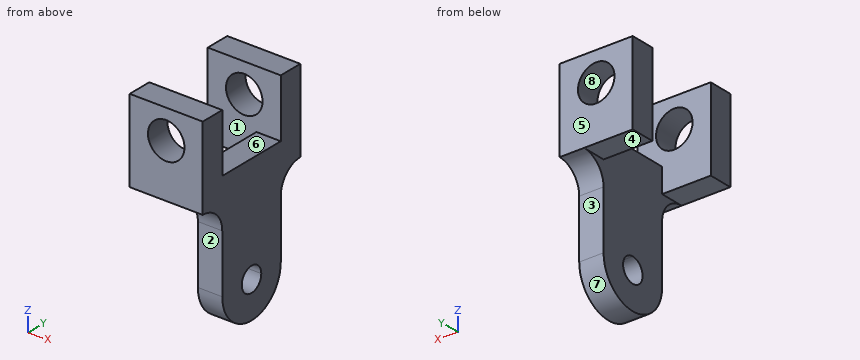
```python
from build123d import *

# Parameters (mm, degrees)
BOSS_EXTRUDE1_DEPTH     = 50
FILLET1_R               = 50
SKETCH2_W               = 150
SKETCH2_H               = 170
BOSS_EXTRUDE2_DEPTH     = 50
SKETCH3_W               = 150
SKETCH3_H               = 170
BOSS_EXTRUDE3_DEPTH     = 50
CUT_EXTRUDE1_DEPTH      = 448.883913531
CUT_EXTRUDE1_DEPTH_BACK = 448.883913531
SKETCH4_R               = 37.5


with BuildPart() as part:
    # Sketch1 → Boss-Extrude1 (new body)
    # profile 1 of 4: a face of its own
    with BuildSketch(Plane.YZ):
        with BuildLine():
            Line((-75, 170), (-75, 0))
            ThreePointArc((-75, 0), (-53.033008589, 53.033008589), (0, 75))
            Line((0, 75), (0, 220))
            Line((0, 220), (-75, 220))
            Line((-75, 220), (-75, 340))
            Line((-75, 340), (-125, 340))
            Line((-125, 340), (-125, 170))
            Line((-125, 170), (-75, 170))
        make_face()
    # profile 2 of 4: a face of its own
    with BuildSketch(Plane.YZ):
        with BuildLine():
            ThreePointArc((0, 75), (53.033008589, 53.033008589), (75, 0))
            Line((75, 0), (75, 170))
            Line((75, 170), (125, 170))
            Line((125, 170), (125, 340))
            Line((125, 340), (75, 340))
            Line((75, 340), (75, 220))
            Line((75, 220), (0, 220))
            Line((0, 220), (0, 75))
        make_face()
    # profile 3 of 4: a face of its own
    with BuildSketch(Plane.YZ):
        with BuildLine():
            ThreePointArc((0, 75), (-53.033008589, 53.033008589), (-75, 0))
            ThreePointArc((-75, 0), (0, -75), (75, 0))
            ThreePointArc((75, 0), (53.033008589, 53.033008589), (0, 75))
        make_face()
        with BuildLine():
            ThreePointArc((25, 0), (-17.67766953, -17.67766953), (0, 25))
            ThreePointArc((0, 25), (17.67766953, 17.67766953), (25, 0))
        make_face(mode=Mode.SUBTRACT)
    # profile 4 of 4: a face of its own
    with BuildSketch(Plane.YZ):
        with BuildLine():
            ThreePointArc((0, 75), (-53.033008589, 53.033008589), (-75, 0))
            ThreePointArc((-75, 0), (0, -75), (75, 0))
            ThreePointArc((75, 0), (53.033008589, 53.033008589), (0, 75))
        make_face()
        with BuildLine():
            ThreePointArc((25, 0), (-17.67766953, -17.67766953), (0, 25))
            ThreePointArc((0, 25), (17.67766953, 17.67766953), (25, 0))
        make_face(mode=Mode.SUBTRACT)
    extrude(amount=-BOSS_EXTRUDE1_DEPTH)

    # Fillet1
    fillet1_edges = [part.edges().sort_by_distance(p)[0] for p in [
        (-25, 75, 170),
        (-25, -75, 170),
    ]]
    fillet(fillet1_edges, radius=FILLET1_R - 0.0001)  # a hair under: the kernel refuses the full size

    # Sketch2 → Boss-Extrude2 (add)
    with BuildSketch(Plane(origin=(0, 125, 0), x_dir=(-1, 0, 0), z_dir=(0, 1, 0))):
        with Locations((75, 255)):
            Rectangle(SKETCH2_W, SKETCH2_H)
    extrude(amount=-BOSS_EXTRUDE2_DEPTH)

    # Sketch3 → Boss-Extrude3 (add)
    with BuildSketch(Plane.XZ.offset(125)):
        with Locations((-75, 255)):
            Rectangle(SKETCH3_W, SKETCH3_H)
    extrude(amount=-BOSS_EXTRUDE3_DEPTH)

    # Sketch4 → Cut-Extrude1 (cut, two sides: drawn at the far end of the back side and taken through both)
    with BuildSketch(Plane.XZ.offset(125).offset(-CUT_EXTRUDE1_DEPTH_BACK)):
        with Locations(Location((-75, 280, 0), (0, 0, 270))):
            Circle(SKETCH4_R)
    extrude(amount=CUT_EXTRUDE1_DEPTH + CUT_EXTRUDE1_DEPTH_BACK, mode=Mode.SUBTRACT)


solid = part.part
```
For this review, take the finished solid that the model builds, in its own axes (mm). Face numbers are marked on the shaded views. A direction names the side the tool comes from. Coordinates: 2 decimals unless noted, no trailing zeros. Loops run counter-clockwise (first coordinate to the right, second up) from the corner with the lowest first, then second, coordinate; pieces in that order, holes last.
1. Add section B-B, the plane x = -75. Give the boundary of the cut face in (y, z).
2. Insertion check: P1, Ø4, axis at x = -35, z = 144.5, coming from the -Y side; P2, Ø12, axis at x = -19.5, y = -12, coming from the -Z side; P3, Ø25, axis at x = -24, z = 45, coming from the +Y side; P4, Ø6, axis at y = -27.5, z = 120.5, coming from the +X side. Each pin has a flat end and moves straight along its axis. Give the tip position at first contact, or say it passes through.
3. For line 1 (X direction, y = 114, z = 280); line 2 (Y direction, x = -120, z = 275); line 3 (Z direction, x = -14, y = 0), list the stretches that pass through material, from the lowest coordinate up.
4. Add section C-C, the plane y = -91. Give the boundary of the cut face in (x, z), then the cut area to 3 significant figures.
5. Mouldability with a two-part tool opening along Y and no side actions: class the marked faces 5, 6, 7 and 8 as +Y half, -Y half, draft (parallel to the pull), parting line (faces both ways), or undercut.
6. Add section D-D, the plane z = 189. Give the boundary of the cut face in (x, y).
7. Add section A-A, the plane z = 280. Give the boundary of the cut face in (x, y), then the cut area to 3 significant figures.
8. For the marked faces 1, 2, 3 and 4, list the 3-axis set-ups (+Z, -Z, +X, -X, +Y, -Y) from which the entire face can be reached by the end or side of a thin tool; tool diameter is ignored.
Result:
1. outline: (-125, 170) - (-75, 170) - (-75, 242.5) - (-125, 242.5) - close; (-125, 317.5) - (-75, 317.5) - (-75, 340) - (-125, 340) - close; (75, 170) - (125, 170) - (125, 242.5) - (75, 242.5) - close; (75, 317.5) - (125, 317.5) - (125, 340) - (75, 340) - close
2. P1: stops at y = -82.6
2. P2: stops at z = -74.76
2. P3: stops at y = 75
2. P4: stops at x = 0
3. line 1: x = -150 to -112.5, -37.5 to 0
3. line 2: y = -125 to -75, 75 to 125
3. line 3: z = -75 to -25, 25 to 220
4. outline: (-150, 170) - (-50, 170) - (-50, 156.66) - (0, 156.66) - (0, 340) - (-150, 340) - close; hole circle Ø75 at (-75, 280)
4. area: 21,700 mm2
5. face 5: +Y half
5. face 6: undercut
5. face 7: parting line
5. face 8: draft
6. outline: (-150, -125) - (0, -125) - (0, 125) - (-150, 125) - (-150, 75) - (-50, 75) - (-50, -75) - (-150, -75) - close
7. outline: (-150, -125) - (-112.5, -125) - (-112.5, -75) - (-150, -75) - close; (-150, 75) - (-112.5, 75) - (-112.5, 125) - (-150, 125) - close; (-37.5, -125) - (0, -125) - (0, -75) - (-37.5, -75) - close; (-37.5, 75) - (0, 75) - (0, 125) - (-37.5, 125) - close
7. area: 7,500 mm2
8. face 1: +Z, -X
8. face 2: -Z, +X, -X, -Y
8. face 3: -Z, +X, -X, +Y
8. face 4: -Z, -X, +Y, -Y
